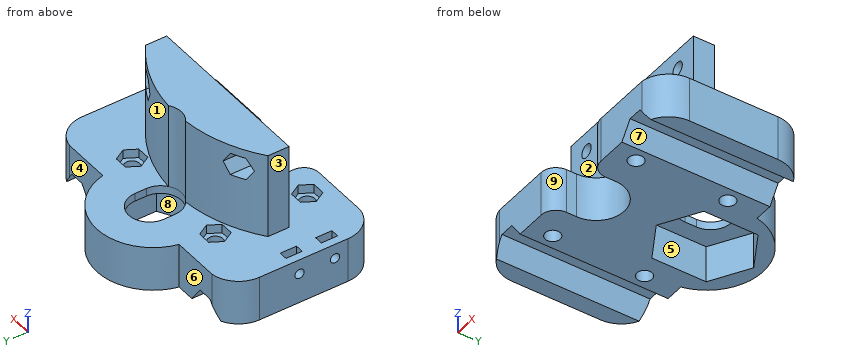
```python
from build123d import *

# Parameters (mm, degrees)
SKETCH1_R                = 2.000043321
SKETCH1_R_2              = 2.000014119
BOSS_EXTRUDE1_DEPTH      = 7.5
BOSS_EXTRUDE1_DEPTH_BACK = 4.5
CUT_EXTRUDE2_DEPTH       = 13
SKETCH3_R                = 2.000014119
SKETCH3_R_2              = 2.000043321
CUT_EXTRUDE3_DEPTH       = 2.38
SKETCH6_W                = 47
SKETCH6_H                = 5.65
BOSS_EXTRUDE2_DEPTH      = 22.75
SKETCH9_R                = 1.8
CUT_EXTRUDE5_DEPTH       = 22.75
CUT_EXTRUDE5_DEPTH_BACK  = 23.750023286
CUT_EXTRUDE6_DEPTH       = 22.75
CUT_EXTRUDE6_DEPTH_BACK  = 4.1004
SKETCH11_R               = 1.250008473
SKETCH11_R_2             = 1.24999389
CUT_EXTRUDE8_DEPTH       = 6.1
SKETCH13_W               = 2.2
SKETCH13_H               = 4.330124
SKETCH13_H_2             = 4.33016
CUT_EXTRUDE9_DEPTH       = 5.3
CUT_EXTRUDE10_DEPTH      = 9.85


with BuildPart() as part:
    # Sketch1 → Boss-Extrude1 (new body, two sides)
    with BuildSketch(Plane.XY) as boss_extrude1_sk:
        with BuildLine():
            ThreePointArc((27.3591, -22.750023286), (32.18573506, -20.04264062), (34.100000001, -14.850154064))
            Line((34.100000001, -14.850154064), (34.100000001, 8.850156137))
            ThreePointArc((34.100000001, 8.850156137), (32.18573506, 14.042642693), (27.3591, 16.750025358))
            Line((27.3591, 16.750025358), (14.6356, 16.750025358))
            ThreePointArc((14.6356, 16.750025358), (0, 28.500025358), (-14.6356, 16.750025358))
            Line((-14.6356, 16.750025358), (-27.3591, 16.750025358))
            ThreePointArc((-27.3591, 16.750025358), (-32.18573506, 14.042642693), (-34.100000001, 8.850156137))
            Line((-34.100000001, 8.850156137), (-34.100000001, -14.850154064))
            ThreePointArc((-34.100000001, -14.850154064), (-32.18573506, -20.04264062), (-27.3591, -22.750023286))
            Line((-27.3591, -22.750023286), (-11.500037792, -22.750023286))
            ThreePointArc((-11.500037792, -22.750023286), (-8.671570628, -21.578433826), (-7.499981167, -18.749966661))
            Line((-7.499981167, -18.749966661), (-7.499981167, -16.089239323))
            ThreePointArc((-7.499981167, -16.089239323), (-7.500113179, -16.044739987), (-7.499981167, -16.000240651))
            ThreePointArc((-7.499981167, -16.000240651), (0, -8.544626807), (7.499981167, -16.000240651))
            ThreePointArc((7.499981167, -16.000240651), (7.500113179, -16.044739987), (7.499981167, -16.089239323))
            Line((7.499981167, -16.089239323), (7.499981167, -18.749966661))
            ThreePointArc((7.499981167, -18.749966661), (8.671570628, -21.578433826), (11.500037792, -22.750023286))
            Line((11.500037792, -22.750023286), (27.3591, -22.750023286))
        make_face()
        with Locations((-16.000068831, -16.5)):
            Circle(SKETCH1_R, mode=Mode.SUBTRACT)
        with Locations((16.000068831, -16.5)):
            Circle(SKETCH1_R, mode=Mode.SUBTRACT)
        with Locations((-16.000068831, 7.999981023)):
            Circle(SKETCH1_R_2, mode=Mode.SUBTRACT)
        with Locations((16.000068831, 7.999981023)):
            Circle(SKETCH1_R_2, mode=Mode.SUBTRACT)
    extrude(amount=BOSS_EXTRUDE1_DEPTH)
    extrude(boss_extrude1_sk.sketch, amount=-BOSS_EXTRUDE1_DEPTH_BACK)

    # Sketch4 → Cut-Extrude2 (cut, through all)
    with BuildSketch(Plane.XY.offset(7.5)):
        with BuildLine():
            Line((5.5, 11.5), (5.5, 14.5))
            ThreePointArc((5.5, 14.5), (0, 20), (-5.5, 14.5))
            Line((-5.5, 14.5), (-5.5, 11.5))
            ThreePointArc((-5.5, 11.5), (0, 6), (5.5, 11.5))
        make_face()
    extrude(amount=-CUT_EXTRUDE2_DEPTH, mode=Mode.SUBTRACT)

    # Sketch3 → Cut-Extrude3 (cut)
    with BuildSketch(Plane.XY.offset(7.5)):
        Polygon((-14.268018024, 10.999981023), (-17.732119639, 10.999981023), (-19.464170446, 7.999981023), (-17.732119639, 4.999981023), (-14.268018024, 4.999981023), (-12.535967216, 7.999981023), align=None)
        with Locations((-16.000068831, 7.999981023)):
            Circle(SKETCH3_R, mode=Mode.SUBTRACT)
        Polygon((14.268018024, 10.999981023), (17.732119639, 10.999981023), (19.464170446, 7.999981023), (17.732119639, 4.999981023), (14.268018024, 4.999981023), (12.535967216, 7.999981023), align=None)
        with Locations((16.000068831, 7.999981023)):
            Circle(SKETCH3_R, mode=Mode.SUBTRACT)
        Polygon((-14.268018024, -19.500018977), (-17.732119639, -19.500018977), (-19.464170446, -16.500018977), (-17.732119639, -13.500018977), (-14.268018024, -13.500018977), (-12.535967216, -16.500018977), align=None)
        with Locations((-16.000068831, -16.5)):
            Circle(SKETCH3_R_2, mode=Mode.SUBTRACT)
        Polygon((12.535967216, -16.500018977), (14.268018024, -19.500018977), (17.732119639, -19.500018977), (19.464170446, -16.500018977), (17.732119639, -13.500018977), (14.268018024, -13.500018977), align=None)
        with Locations((16.000068831, -16.5)):
            Circle(SKETCH3_R_2, mode=Mode.SUBTRACT)
    extrude(amount=-CUT_EXTRUDE3_DEPTH, mode=Mode.SUBTRACT)

    # Sketch6 → Boss-Extrude2 (add)
    with BuildSketch(Plane.XY.offset(7.5)):
        with Locations((0, -3.625)):
            Rectangle(SKETCH6_W, SKETCH6_H)
        with BuildLine():
            Line((-23.5, -0.8), (23.5, -0.8))
            ThreePointArc((23.5, -0.8), (13.984131025, 4.616883926), (3.324005419, 7.118106805))
            ThreePointArc((3.324005419, 7.118106805), (0, 6), (-3.324005419, 7.118106805))
            ThreePointArc((-3.324005419, 7.118106805), (-13.984131025, 4.616883926), (-23.5, -0.8))
        make_face()
    extrude(amount=BOSS_EXTRUDE2_DEPTH)

    # Sketch9 → Cut-Extrude5 (cut, two sides)
    with BuildSketch(Plane(origin=(0, 0, 0), x_dir=(1, 0, 0), z_dir=(0, 1, 0))) as cut_extrude5_sk:
        Polygon((19.555132158, 4.5), (22.70606608, 0), (26.49606608, 0), (29.647000001, 4.5), align=None)
        Polygon((-19.555132158, 4.5), (-29.647000001, 4.5), (-26.49606608, 0), (-22.70606608, 0), align=None)
        with Locations((17.5, -25)):
            Circle(SKETCH9_R)
        with Locations((-17.5, -25)):
            Circle(SKETCH9_R)
    extrude(amount=CUT_EXTRUDE5_DEPTH, mode=Mode.SUBTRACT)
    extrude(cut_extrude5_sk.sketch, amount=-CUT_EXTRUDE5_DEPTH_BACK, mode=Mode.SUBTRACT)

    # Sketch9_7 → Cut-Extrude6 (cut, two sides)
    with BuildSketch(Plane(origin=(0, 0, 0), x_dir=(1, 0, 0), z_dir=(0, 1, 0))) as cut_extrude6_sk:
        Polygon((-19.232050808, -22), (-20.964101615, -25), (-19.232050808, -28), (-15.767949192, -28), (-14.035898385, -25), (-15.767949192, -22), align=None)
        Polygon((20.964101615, -25), (19.232050808, -28), (15.767949192, -28), (14.035898385, -25), (15.767949192, -22), (19.232050808, -22), align=None)
    extrude(amount=CUT_EXTRUDE6_DEPTH, mode=Mode.SUBTRACT)
    extrude(cut_extrude6_sk.sketch, amount=-CUT_EXTRUDE6_DEPTH_BACK, mode=Mode.SUBTRACT)

    # Sketch11 → Cut-Extrude8 (cut)
    with BuildSketch(Plane.ZY.offset(34.100000001)):
        with Locations((3.549979666, -1.86999177)):
            Circle(SKETCH11_R)
        with Locations((3.549979666, -11.329991983)):
            Circle(SKETCH11_R_2)
    extrude(amount=-CUT_EXTRUDE8_DEPTH, mode=Mode.SUBTRACT)

    # Sketch13 → Cut-Extrude9 (cut)
    with BuildSketch(Plane.XY.offset(7.5)):
        with Locations((-30.9, -1.869998)):
            Rectangle(SKETCH13_W, SKETCH13_H)
        with Locations((-30.9, -11.33002)):
            Rectangle(SKETCH13_W, SKETCH13_H_2)
    extrude(amount=-CUT_EXTRUDE9_DEPTH, mode=Mode.SUBTRACT)

    # Sketch15 → Cut-Extrude10 (cut)
    with BuildSketch(Plane(origin=(0, 0, -4.5), x_dir=(-1, 0, 0), z_dir=(0, 0, -1))):
        Polygon((-7.2e-08, 26), (-9.95929, 20.25), (-9.95929, 5.75), (7.2e-08, 1.24e-07), (9.95929, 5.75), (9.95929, 20.25), align=None)
    extrude(amount=-CUT_EXTRUDE10_DEPTH, mode=Mode.SUBTRACT)


solid = part.part
```
Verification items for the finished model (mm, model axes). Face numbers are marked on the shaded views. A direction names the side the tool comes from. Coordinates: 2 decimals unless noted, no trailing zeros. Loops run counter-clockwise (first coordinate to the right, second up) from the corner with the lowest first, then second, coordinate; pieces in that order, holes last. Notation, with made-up numbers: (11.5, 14.5) - (36.5, 14.5) arc R10 ccw to (36.5, 20.5) - close; hole circle Ø8 at (46, -10). An arc over 180 degrees is marked (long way). Answer as a JSON object with one key per item and string values.
(1) Cross-section at B-B, the plane x = -9. Record the boundary of the cut face in (y, z).
Response:
{"outline": "(-21.87, -4.5) - (5.2, -4.5) - (5.2, 5.35) - (20.8, 5.35) - (20.8, -4.5) - (25.5, -4.5) - (25.5, 7.5) - (6.19, 7.5) - (6.19, 30.25) - (-6.45, 30.25) - (-6.45, 7.5) - (-21.87, 7.5) - close"}
(2) Scan lines: line 1 along X through (y, z) = (-5.1, 25); line 2 along X through (y, z) = (-16, 7); line 3 along Z through (x, y) = (17.5, -4.55). Record each from-to range of solid material in increasing order.
Response:
{"line 1": "x = -23.5 to -19.3, -15.7 to 15.7, 19.3 to 23.5", "line 2": "x = -34.02 to -19.18, -12.82 to -7.5, 7.5 to 12.82, 19.18 to 34.02", "line 3": "z = -4.5 to 23.2, 26.8 to 30.25"}
(3) Cross-section at D-D, the plane x = 6.5. Record the boundary of the cut face in (y, z).
Response:
{"outline": "(-12.3, -4.5) - (3.75, -4.5) - (3.75, 5.35) - (22.25, 5.35) - (22.25, -4.5) - (27.02, -4.5) - (27.02, 7.5) - (6.71, 7.5) - (6.71, 30.25) - (-6.45, 30.25) - (-6.45, 7.5) - (-12.3, 7.5) - close"}
(4) Mould release check, pull along Y, two halves, no side actions. Record for the marked faces 6, 7, 8 and 9: pulls with the +Y half, pulls with the -Y half, needs draft (parallel to the pull), parting line crosses it, or undercut.
Response:
{"face 6": "pulls with the +Y half", "face 7": "needs draft", "face 8": "undercut", "face 9": "pulls with the -Y half"}
(5) Go/stop test with flat-tipped pins: pin 1 Ø1.1 at (x, z) = (-31.5, 6) entering from -Y; pin 2 Ø12 at (y, z) = (-8, 18.5) entering from +X; pin 3 Ø3 at (x, z) = (-1.5, 16.5) entering from +Y. Record where each tip stops, or that it passes through.
Response:
{"pin 1": "stops at y = -21.21", "pin 2": "stops at x = 23.5", "pin 3": "stops at y = 6.89"}
(6) Cross-section at C-C, the plane y = 22.5. Record the boundary of the cut face in (x, z).
Response:
{"outline": "(-11.99, -4.5) - (-6.06, -4.5) - (-6.06, 5.35) - (6.06, 5.35) - (6.06, -4.5) - (11.99, -4.5) - (11.99, 7.5) - (-11.99, 7.5) - close"}
(7) Cross-section at A-A, the plane z = 15.5. Record the boundary of the cut face in (x, y), then the cut area to 3 significant figures.
Response:
{"outline": "(-23.5, -6.45) - (23.5, -6.45) - (23.5, -0.8) arc R38.28 ccw to (3.32, 7.12) arc R5.5 cw to (-3.32, 7.12) arc R38.28 ccw to (-23.5, -0.8) - close", "area": "518 mm²"}
(8) Access from +Z, -Z, +X, -X, +Y, -Y to the whole of each face (thin tool, end or side, straight path). Record for the marked faces 1, 2, 3, 4 and 5.
Response:
{"face 1": "+Z, +X, +Y", "face 2": "+Z, +X, -X, -Y", "face 3": "+Z, -X, +Y, -Y", "face 4": "+Z, -Z, +X, +Y", "face 5": "-Z"}
